Geometry: final body of the model. Coordinates: model frame, mm. A direction names the side the tool comes from. Round coordinates to 2 decimals unless told otherwise and drop trailing zeros. Loops run counter-clockwise (first coordinate to the right, second up) from the corner with the lowest first, then second, coordinate; pieces in that order, holes last. Notation, with made-up numbers: (68.25, -14.75) - (118.25, -14.75) arc R10 ccw to (118.25, 2.25) - close; hole circle Ø6 at (8.25, 54). An arc over 180 degrees is marked (long way). Answer as a JSON object with one key per item and string values. Group by question number.
Item 1: Reachability of faces 5 (the face through (45, 2, 5.3)), 6 (the face through (1.846, -41.451, 3.88)) from +Z, -Z, +X, -X, +Y, -Y: full face, straight path, thin tool, end or side. Return the list, or none.
Item 2: Line query: line 1 (Y direction, x = 0, z = 3.45); line 2 (X direction, y = -45, z = 3); line 3 (Z direction, x = -16, y = 26). Output: solid intervals per line, ascending.
Item 3: Draft query along X for faces 1 (the face through (-0.18, -46.39, 2.61)), 2 (the face through (-11.923, -53.692, 1.232)), 3 (the face through (0, 47, 5.3)), 4 (the face through (46.335, -0.421, 2.613)). Return one class per face: released by +X, released by -X, zero draft, split by the parting line, or undercut.
Item 4: Section A-A (y = 0). Return the cut outline in (x, z).
Item 5: Section C-C (y = -45). Return the cut outline in (x, z), plus the area to 3 significant figures.
Item 6: First-contact query: pin 1 (3.5 mm diameter, centred on x = -45, y = 0, fed in from -Z); pin 2 (2 mm diameter, centred on y = -27, z = 3, fed in from -X); pin 3 (3 mm diameter, centred on x = 40, z = 0.5, fed in from -Y); pin 4 (10 mm diameter, centred on x = 35, y = 10.5, fed in from +Z). Flat tips, straight axial feed; report the tip coordinate or a pass-through.
```python
from build123d import *

# Parameters (mm, degrees)
F0_R     = 55
F1_DEPTH = 2.5
F2_R     = 1.4
F3_DEPTH = 12.5
F2_R_2   = 4
F4_DEPTH = 5.3


with BuildPart() as f1:
    # F0 (on Top) → F1 (new body)
    with BuildSketch(Plane.XY):
        Circle(F0_R)
    extrude(amount=F1_DEPTH)

    # F2 (on face) → F3 (cut, symmetric)
    with BuildSketch(Plane(origin=(0, 0, 0), x_dir=(1, 0, 0), z_dir=(0, 0, -1))):
        with Locations((0, -45)):
            Circle(F2_R)
        with Locations((-45, 0)):
            Circle(F2_R)
        with Locations((0, 45)):
            Circle(F2_R)
        with Locations((45, 0)):
            Circle(F2_R)
    extrude(amount=F3_DEPTH, both=True, mode=Mode.SUBTRACT)

    # F2 (on face) → F4 (join)
    with BuildSketch(Plane(origin=(0, 0, 0), x_dir=(1, 0, 0), z_dir=(0, 0, -1))):
        with Locations((-45, 0)):
            Circle(F2_R_2)
        with Locations((-45, 0)):
            Circle(F2_R, mode=Mode.SUBTRACT)
        with Locations((0, -45)):
            Circle(F2_R_2)
        with Locations((0, -45)):
            Circle(F2_R, mode=Mode.SUBTRACT)
        with Locations((45, 0)):
            Circle(F2_R_2)
        with Locations((45, 0)):
            Circle(F2_R, mode=Mode.SUBTRACT)
        with Locations((0, 45)):
            Circle(F2_R_2)
        with Locations((0, 45)):
            Circle(F2_R, mode=Mode.SUBTRACT)
    extrude(amount=-F4_DEPTH)


solid = f1.part
```
Values:
{
 "1": {"face 5": "+Z, +X, -X, +Y, -Y", "face 6": "+Z"},
 "2": {"line 1": "y = -49 to -46.4, -43.6 to -41, 41 to 43.6, 46.4 to 49", "line 2": "x = -4 to -1.4, 1.4 to 4", "line 3": "z = 0 to 2.5"},
 "3": {"face 1": "undercut", "face 2": "split by the parting line", "face 3": "zero draft", "face 4": "undercut"},
 "4": {"outline": "(-55, 0) - (-46.4, 0) - (-46.4, 5.3) - (-49, 5.3) - (-49, 2.5) - (-55, 2.5) - close; (-43.6, 0) - (43.6, 0) - (43.6, 5.3) - (41, 5.3) - (41, 2.5) - (-41, 2.5) - (-41, 5.3) - (-43.6, 5.3) - close; (46.4, 0) - (55, 0) - (55, 2.5) - (49, 2.5) - (49, 5.3) - (46.4, 5.3) - close"},
 "5": {"outline": "(-31.62, 0) - (-1.4, 0) - (-1.4, 5.3) - (-4, 5.3) - (-4, 2.5) - (-31.62, 2.5) - close; (1.4, 0) - (31.62, 0) - (31.62, 2.5) - (4, 2.5) - (4, 5.3) - (1.4, 5.3) - close", "area": "166 mm^2"},
 "6": {"pin 1": "stops at z = 0", "pin 2": "stops at x = -48.39", "pin 3": "stops at y = -39.28", "pin 4": "stops at z = 2.5"}
}
